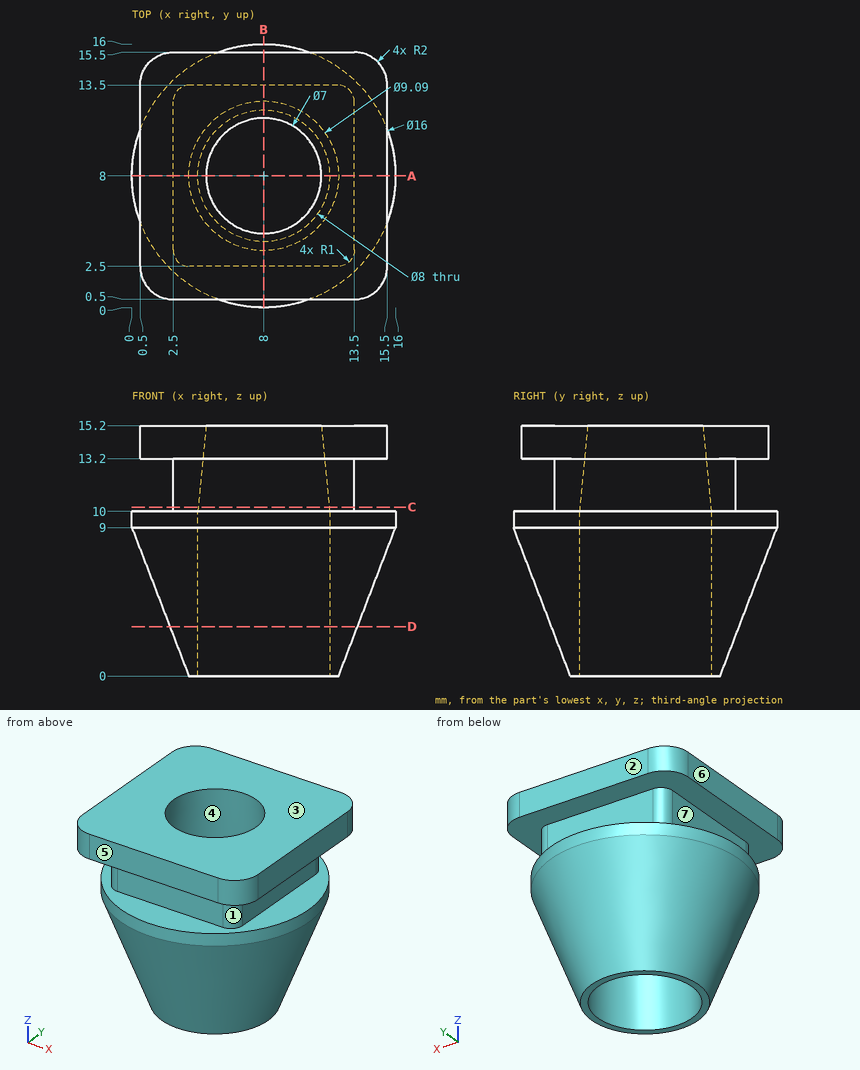
Study the drawing (mm; zero at the part's minimum x, y, z) and answer. A direction names the side the tool comes from. Coordinates: 2 decimals unless noted, no trailing zeros. Write each loop counter-clockwise with the first axis right and the second up, starting at its lowest first coordinate (ties: lowest second). Pieces come first, ordered by that corner, then holes. Notation, with made-up numbers: M -27.5,4 L 6.5,4 A11 ccw 6.5,10 Z; hole C 12.25,-26 d1. An arc over 180 degrees is marked long. Use a Markdown table: item, result. Add a question column.
1. Section C-C (z = 10.25) is taken. Give the vertices of the cut face in (x, y).
2. For a pull along Y with two mould halves and no side action, classify the marked faces 1, 2, 3 and 4 as +Y half, -Y half, draft (parallel to the pull), parting line (faces both ways), or undercut.
3. Which of the six approach directions +Z, -Z, +X, -X, +Y, -Y give full straight-line access (tool end or side, diameter ignored) to the marked faces 5, 6 and 7?
4. Straight lines are drawn through the part: line 1 along Y through (x, z) = (10.75, 11.5) (1 decimal); line 2 along Y through (x, z) = (8, 10.75); line 3 along Z through (x, y) = (5.5, 14.5) (1 decimal). For each, find the intervals that lie inside material, in ascending order. Write a range as [from, to].
5. Section A-A (y = 8) is taken. Give the vertices of the cut face in (x, z) (1 decimal).
6. Given P1, Ø1.6, axis at y = 6.5, z = 11, coming from the +X side; P2, Ø3.5, axis at x = 9.5, z = 12, coming from the +Y side; P3, Ø5, axis at x = 3, z = 10.5, coming from the +Y side, each flat-ended and moving along its own axis, determine where each tip first touches the part or whether it passes through.
7. Section D-D (z = 3) is taken. Give the vertices of the cut face in (x, y).
Data:
| question | item | result |
|---|---|---|
| 1 | outline | M 2.5,3.5 A1 ccw 3.5,2.5 L 12.5,2.5 A1 ccw 13.5,3.5 L 13.5,12.5 A1 ccw 12.5,13.5 L 3.5,13.5 A1 ccw 2.5,12.5 Z; hole C 8,8 d7.95 |
| 2 | face 1 | -Y half |
| 2 | face 2 | +Y half |
| 2 | face 3 | draft |
| 2 | face 4 | undercut |
| 3 | face 5 | +Z, +X, -X, -Y |
| 3 | face 6 | +Z, -X, +Y, -Y |
| 3 | face 7 | -X, +Y, -Y |
| 4 | line 1 | y = [2.5, 5.3], [10.7, 13.5] |
| 4 | line 2 | y = [2.5, 4.07], [11.93, 13.5] |
| 4 | line 3 | z = [6.3, 10], [13.2, 15.2] |
| 5 | outline | M 0,9 L 3.5,0 L 4,0 L 4,10 L 4.5,15.2 L 0.5,15.2 L 0.5,13.2 L 2.5,13.2 L 2.5,10 L 0,10 Z; M 11.5,15.2 L 12,10 L 12,0 L 12.5,0 L 16,9 L 16,10 L 13.5,10 L 13.5,13.2 L 15.5,13.2 L 15.5,15.2 Z |
| 6 | P1 | stops at x = 13.5 |
| 6 | P2 | stops at y = 15.5 |
| 6 | P3 | stops at y = 15.58 |
| 7 | outline | C 8,8 d11.39; hole C 8,8 d8 |
